```python
from build123d import *

# Parameters (mm, degrees)
SKETCH_1_W          = 71
SKETCH_1_H          = 30
SKETCH_1_R          = 1.5
EXTRUDE_1_DEPTH     = 4
FILLET_1_R          = 3
SKETCH_3_W          = 4.5
SKETCH_3_H          = 30
EXTRUDE_3_DEPTH     = 32
SKETCH_4_R          = 1.25
SKETCH_4_R_2        = 12
CUT_EXTRUDE_1_DEPTH = 30
FILLET_2_R          = 3
FILLET_3_R          = 1


with BuildPart() as part:
    # 草图1 → 凸台-拉伸1 (new body)
    with BuildSketch(Plane(origin=(0, 0, 0), x_dir=(1, 0, 0), z_dir=(0, 1, 0))):
        Rectangle(SKETCH_1_W, SKETCH_1_H)
        with Locations(Location((31.6, 11, 0), (0, 0, 270))):
            Circle(SKETCH_1_R, mode=Mode.SUBTRACT)
        with Locations(Location((31.6, 3, 0), (0, 0, 90))):
            Circle(SKETCH_1_R, mode=Mode.SUBTRACT)
        with Locations(Location((-31.6, 3, 0), (0, 0, 270))):
            Circle(SKETCH_1_R, mode=Mode.SUBTRACT)
        with Locations(Location((-31.6, 11, 0), (0, 0, 90))):
            Circle(SKETCH_1_R, mode=Mode.SUBTRACT)
    extrude(amount=EXTRUDE_1_DEPTH)

    # 圆角1
    fillet_1_edges = [part.edges().sort_by_distance(p)[0] for p in [
        (35.5, 2, 15),
        (-35.5, 2, 15),
        (-35.5, 2, -15),
        (35.5, 2, -15),
    ]]
    fillet(fillet_1_edges, radius=FILLET_1_R)

    # 草图3 → 凸台-拉伸3 (add)
    with BuildSketch(Plane.XZ):
        with Locations((-24.75, 0)):
            Rectangle(SKETCH_3_W, SKETCH_3_H)
    extrude(amount=EXTRUDE_3_DEPTH)

    # 草图4 → 切除-拉伸1 (cut)
    with BuildSketch(Plane.ZY.offset(27)):
        with Locations((11.5, -4.5)):
            Circle(SKETCH_4_R)
        with Locations((11.5, -27.5)):
            Circle(SKETCH_4_R)
        with Locations((-11.5, -27.5)):
            Circle(SKETCH_4_R)
        with Locations((-11.5, -4.5)):
            Circle(SKETCH_4_R)
        with Locations((0, -16)):
            Circle(SKETCH_4_R_2)
    extrude(amount=-CUT_EXTRUDE_1_DEPTH, mode=Mode.SUBTRACT)

    # 圆角2
    fillet_2_edges = [part.edges().sort_by_distance(p)[0] for p in [
        (-24.75, -32, -15),
        (-24.75, -32, 15),
    ]]
    fillet(fillet_2_edges, radius=FILLET_2_R)

    # 圆角3
    fillet_3_edges = [part.edges().sort_by_distance(p)[0] for p in [
        (-22.5, 0, 0),
    ]]
    fillet(fillet_3_edges, radius=FILLET_3_R)


solid = part.part
```
Source: CAD feature listing. Evaluate the final solid. Frame: model axes, mm. A direction names the side the tool comes from. Coordinates: 2 decimals unless noted, no trailing zeros. Loops run counter-clockwise (first coordinate to the right, second up) from the corner with the lowest first, then second, coordinate; pieces in that order, holes last. Notation, with made-up numbers: M 59.5,46.25 L 63.5,46.25 A7 cw 63.5,50.25 Z; hole C 51,40.25 d4. An arc over 180 degrees is marked long. Use a Markdown table: item, result. Add a question column.
Q1. Access query for faces 5 (the flat face through (7, 0, 0)), 6 (the cylindrical face through (-24.78, -27.45, -12.75)). Directions: +Z, -Z, +X, -X, +Y, -Y. A direction counts if a zero-diameter tool reaches every point of the face in a straight line with its end or side. Return the directions, or none.
Q2. Material intervals for L1, parallel to Z at x = -25, y = -27; L2, parallel to X at y = 1.5, z = -12.25; L3, parallel to X at y = -5, z = -7.5, sorted ascending.
Q3. Section query D-D, the plane y = -2.5. Return loops of the section in (x, z), and give its area (3 significant figures).
Q4. Draft query along Y for faces 1 (the cylindrical face through (-24.78, -4.1, -1.56)), 2 (the flat face through (-31, 0, 0)), 3 (the cylindrical face through (-24.78, -5.26, 10.51)), 4 (the cylindrical face through (34.6, 2.03, -14.14)). Return one class per face: pulls with the +Y half, pulls with the -Y half, needs draft (parallel to the pull), parting line crosses it, or undercut.
Q5. First-contact query: pin 1 (3 mm diameter, centred on y = -4.5, z = 11.5, fed in from +X); pin 2 (2.5 mm diameter, centred on x = 31.6, z = -11, fed in from -Y); pin 3 (5 mm diameter, centred on x = 21.5, z = -3, fed in from -Y); pin 4 (3 mm diameter, centred on y = -4.5, z = -11.5, fed in from -X). Flat tips, straight axial feed; report the tip coordinate or a pass-through.
Q6. Section query C-C, the plane z = 4.5. Return loops of the section in (x, y), and give its area (3 significant figures).
Q7. Section query A-A, the plane x = -31.6. Return loops of the section in (y, z), and give its area (3 significant figures).
Q8. Section query B-B, the plane y = -25. Return loops of the section in (x, z), and give its area (3 significant figures).
Result:
| question | item | result |
|---|---|---|
| 1 | face 5 | +Z, -Z, +X, -Y |
| 1 | face 6 | +X, -X |
| 2 | L1 | z = -15 to -12.65, -10.35 to -4.8, 4.8 to 10.35, 12.65 to 15 |
| 2 | L2 | x = -35.49 to -32.43, -30.77 to 30.77, 32.43 to 35.49 |
| 2 | L3 | x = -27 to -22.5 |
| 3 | outline | M -27,-15 L -22.5,-15 L -22.5,15 L -27,15 Z |
| 3 | area | 135 mm2 |
| 4 | face 1 | undercut |
| 4 | face 2 | pulls with the -Y half |
| 4 | face 3 | undercut |
| 4 | face 4 | needs draft |
| 5 | pin 1 | stops at x = -22.5 |
| 5 | pin 2 | passes through |
| 5 | pin 3 | stops at y = 0 |
| 5 | pin 4 | stops at x = -27 |
| 6 | outline | M -35.5,0 L -27,0 L -27,-4.88 L -22.5,-4.88 L -22.5,-1 A1 cw -21.5,0 L 35.5,0 L 35.5,4 L -35.5,4 Z; M -27,-32 L -22.5,-32 L -22.5,-27.12 L -27,-27.12 Z |
| 6 | area | 328 mm2 |
| 7 | outline | M 0,-15 L 4,-15 L 4,-12.5 L 0,-12.5 Z; M 0,-9.5 L 4,-9.5 L 4,-4.5 L 0,-4.5 Z; M 0,-1.5 L 4,-1.5 L 4,15 L 0,15 Z |
| 7 | area | 96.0 mm2 |
| 8 | outline | M -27,-15 L -22.5,-15 L -22.5,-7.94 L -27,-7.94 Z; M -27,7.94 L -22.5,7.94 L -22.5,15 L -27,15 Z |
| 8 | area | 63.6 mm2 |
